Can you work these out from the drawing? Everything is in mm from the part's minimum corner. A direction names the side the tool comes from. Give positions to 0.01 mm unless a question says otherwise; leave off trailing zeros. Order: outer loops, then holes, each group sorted by start corner. A loop starts at its lowest first (then second) coordinate and runs counter-clockwise, first axis right, second up. Notation, with made-up numbers: (0.25, -34) -> (55.25, -34) arc R29 cw to (55.25, 0) -> close; hole circle Ø5 at (46, 4.25). An arc over 180 degrees is marked (long way). One line per item, written item: value.
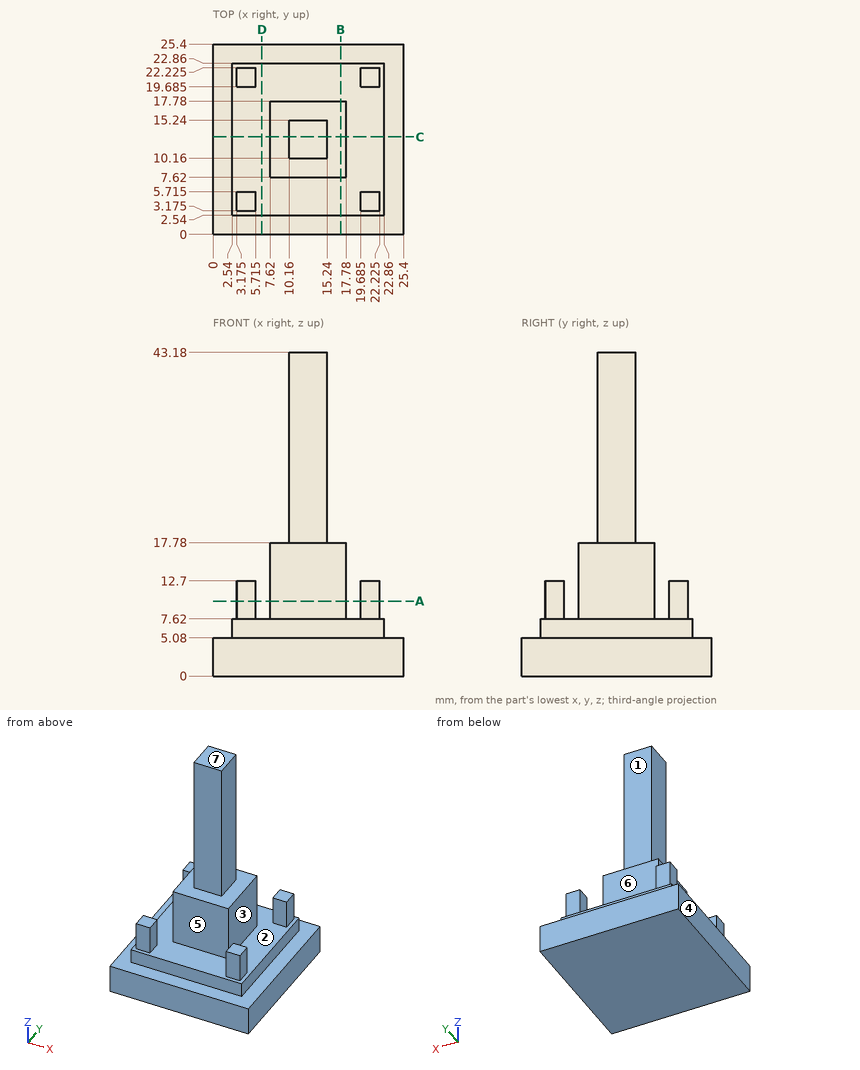
1) Suppose I cut it at A-A, the plane z = 10. Write out the boundary of the cut face in (x, y) (3 decimals).
Answer below:
outline: (3.175, 3.175) -> (5.715, 3.175) -> (5.715, 5.715) -> (3.175, 5.715) -> close; (3.175, 19.685) -> (5.715, 19.685) -> (5.715, 22.225) -> (3.175, 22.225) -> close; (7.62, 7.62) -> (17.78, 7.62) -> (17.78, 17.78) -> (7.62, 17.78) -> close; (19.685, 3.175) -> (22.225, 3.175) -> (22.225, 5.715) -> (19.685, 5.715) -> close; (19.685, 19.685) -> (22.225, 19.685) -> (22.225, 22.225) -> (19.685, 22.225) -> close
2) Suppose I cut it at D-D, the plane x = 6.5. Write out the boundary of the cut face in (y, z).
Answer below:
outline: (0, 0) -> (25.4, 0) -> (25.4, 5.08) -> (22.86, 5.08) -> (22.86, 7.62) -> (2.54, 7.62) -> (2.54, 5.08) -> (0, 5.08) -> close
3) For the marked faces 5, 6 and 7, which set-ups out of +Z, -Z, +X, -X, +Y, -Y let a thin tool reach every point of the face, with its end or its side?
Answer below:
face 5: +Z, +X, -X, -Y
face 6: +Z, +X, -X, +Y
face 7: +Z, +X, -X, +Y, -Y
4) If I drill on line 1 along Y through (x, z) = (10.75, 27.5); line 2 along Z through (x, y) = (11.25, 2); line 3 along Z through (x, y) = (22.5, 18.75), over which ranges is the centre line in solid material (lowest first)?
Answer below:
line 1: y = 10.16 to 15.24
line 2: z = 0 to 5.08
line 3: z = 0 to 7.62
5) For P1, Ø2.5, axis at y = 12, z = 31, coming from the +X side; P2, Ø1.3, axis at x = 4.5, z = 9, coming from the -Y side (3 decimals); P3, Ø5, axis at y = 12.5, z = 24, coming from the -X side, each with a flat end and sliding along its axis, tell me the tip position at first contact or that it passes through.
Answer below:
P1: stops at x = 15.24
P2: stops at y = 3.175
P3: stops at x = 10.16
6) We'd pull the mould along X, two halves only. Please class the marked faces 1, 2, 3 and 4: +X half, -X half, draft (parallel to the pull), parting line (faces both ways), or undercut.
Answer below:
face 1: draft
face 2: undercut
face 3: +X half
face 4: -X half
7) Suppose I cut it at C-C, the plane y = 13. Write out the boundary of the cut face in (x, z), then the cut area to 3 significant figures.
Answer below:
outline: (0, 0) -> (25.4, 0) -> (25.4, 5.08) -> (22.86, 5.08) -> (22.86, 7.62) -> (17.78, 7.62) -> (17.78, 17.78) -> (15.24, 17.78) -> (15.24, 43.18) -> (10.16, 43.18) -> (10.16, 17.78) -> (7.62, 17.78) -> (7.62, 7.62) -> (2.54, 7.62) -> (2.54, 5.08) -> (0, 5.08) -> close
area: 413 mm2
8) Suppose I cut it at B-B, the plane x = 17. Write out the boundary of the cut face in (y, z), then the cut area to 3 significant figures.
Answer below:
outline: (0, 0) -> (25.4, 0) -> (25.4, 5.08) -> (22.86, 5.08) -> (22.86, 7.62) -> (17.78, 7.62) -> (17.78, 17.78) -> (7.62, 17.78) -> (7.62, 7.62) -> (2.54, 7.62) -> (2.54, 5.08) -> (0, 5.08) -> close
area: 284 mm2
